Could you check a few things on this model? Use its own coordinates, in mm. A direction names the side the tool comes from. Round coordinates to 2 decimals unless told otherwise and drop trailing zeros. Loops run counter-clockwise (first coordinate to the right, second up) from the corner with the lowest first, then second, coordinate; pieces in that order, holes last. Notation, with made-up numbers: M -36,64.5 L -24,64.5 A22 cw -24,81.5 Z; hole C 11,37.5 d1. An arc over 180 degrees is marked long. One line per item, written item: value. Start each with the question number.
Q1. I'm going to push flat-ended pins straight in: pin 1 Ø1 at (x, z) = (1, -51.5) entering from +Y; pin 2 Ø1.5 at (x, z) = (2, -55.5) entering from -Y. Where does each tip first touch, or does it pass through?
Q2. Imagine slicing it at D-D (z = -45). Please give me the cut outline in (x, y).
Q3. Which directions (+Z, -Z, +X, -X, +Y, -Y) give clear straight access to the entire face, cutting with the end or side of a thin tool? Please do faces 4 (the face through (1, 20, -45)), 5 (the face through (1, 0, -72.35)), 6 (the face through (1, -23, -22)), 7 (the face through (1, -20, -45)), 8 (the face through (1.52, 0.18, -21.1)).
Q4. Imagine slicing it at B-B (x = 0.55). Please give me the cut outline in (y, z), then the cut area to 3 significant figures.
Q5. Imagine slicing it at C-C (y = 0). Please give me the cut outline in (x, z), then the cut area to 3 significant figures.
Q6. Thinking about a two-plate mould opening in Y: for faces 1 (the face through (1, 0, 27.45)), 2 (the face through (1, 23, -22)), 3 (the face through (2, 8.1, 0)), which applies, released by +Y, released by -Y, zero draft, split by the parting line, or undercut?
Q7. Please list where these lines run through material, in increasing order: line 1 along Y through (x, z) = (1.95, 20.5); line 2 along Z through (x, y) = (2.4, 8.5); line 3 along Y through (x, z) = (2.5, -6.5).
Q8. Imagine slicing it at A-A (z = -4). Please give me the cut outline in (x, y).
from build123d import *

# Parameters (mm, degrees)
SKETCH1_W           = 99.8
SKETCH1_H           = 40
SKETCH1_W_2         = 10
SKETCH1_H_2         = 3
BOSS_EXTRUDE1_DEPTH = 3
SKETCH2_R           = 1.1
CUT_EXTRUDE1_DEPTH  = 76.977118266


with BuildPart() as part:
    # Sketch1 → Boss-Extrude1 (new body)
    with BuildSketch(Plane(origin=(0, 0, 0), x_dir=(0, 0, -1), z_dir=(1, 0, 0))):
        with Locations((22.45, 0)):
            Rectangle(SKETCH1_W, SKETCH1_H)
        with Locations((-22.45, 21.5)):
            Rectangle(SKETCH1_W_2, SKETCH1_H_2)
        with Locations((22.45, 21.5)):
            Rectangle(SKETCH1_W_2, SKETCH1_H_2)
        with Locations((67.35, 21.5)):
            Rectangle(SKETCH1_W_2, SKETCH1_H_2)
        with Locations((67.35, -21.5)):
            Rectangle(SKETCH1_W_2, SKETCH1_H_2)
        with Locations((22.45, -21.5)):
            Rectangle(SKETCH1_W_2, SKETCH1_H_2)
        with Locations((-22.45, -21.5)):
            Rectangle(SKETCH1_W_2, SKETCH1_H_2)
    extrude(amount=BOSS_EXTRUDE1_DEPTH)

    # Sketch2 → Cut-Extrude1 (cut, through all)
    with BuildSketch(Plane(origin=(3, 0, 0), x_dir=(0, 0, -1), z_dir=(1, 0, 0))):
        with Locations((-20.5, 8)):
            Circle(SKETCH2_R)
        with Locations((-20.5, -8)):
            Circle(SKETCH2_R)
        with Locations((20.5, 8)):
            Circle(SKETCH2_R)
        with Locations((20.5, -8)):
            Circle(SKETCH2_R)
        with BuildLine():
            Line((-13, 8.1), (13, 8.1))
            ThreePointArc((13, 8.1), (21.1, 0), (13, -8.1))
            Line((13, -8.1), (-13, -8.1))
            ThreePointArc((-13, -8.1), (-21.1, 0), (-13, 8.1))
        make_face()
    extrude(amount=-CUT_EXTRUDE1_DEPTH, mode=Mode.SUBTRACT)


solid = part.part
Report:
1. pin 1: stops at y = 20
1. pin 2: stops at y = -20
2. outline: M 0,-20 L 3,-20 L 3,20 L 0,20 Z
3. face 4: +X, -X, +Y
3. face 5: -Z, +X, -X, +Y, -Y
3. face 6: +Z, -Z, +X, -X, -Y
3. face 7: +X, -X, -Y
3. face 8: +X, -X
4. outline: M -23,-72.35 L 23,-72.35 L 23,-62.35 L 20,-62.35 L 20,-27.45 L 23,-27.45 L 23,-17.45 L 20,-17.45 L 20,17.45 L 23,17.45 L 23,27.45 L -23,27.45 L -23,17.45 L -20,17.45 L -20,-17.45 L -23,-17.45 L -23,-27.45 L -20,-27.45 L -20,-62.35 L -23,-62.35 Z; hole C -8,-20.5 d2.2; hole C -8,20.5 d2.2; hole M -8.1,-13 A8.1 ccw 8.1,-13 L 8.1,13 A8.1 ccw -8.1,13 Z; hole C 8,-20.5 d2.2; hole C 8,20.5 d2.2
4. area: 3,530 mm²
5. outline: M 0,-72.35 L 3,-72.35 L 3,-21.1 L 0,-21.1 Z; M 0,21.1 L 3,21.1 L 3,27.45 L 0,27.45 Z
5. area: 173 mm²
6. face 1: zero draft
6. face 2: released by +Y
6. face 3: undercut
7. line 1: y = -23 to -9.1, -6.9 to -3.06, 3.06 to 6.9, 9.1 to 23
7. line 2: z = -72.35 to -21.48, -19.52 to 19.52, 21.48 to 27.45
7. line 3: y = -20 to -8.1, 8.1 to 20
8. outline: M 0,-20 L 3,-20 L 3,-8.1 L 0,-8.1 Z; M 0,8.1 L 3,8.1 L 3,20 L 0,20 Z
